The listing builds one solid part. Answer for the finished solid, in the listing's coordinates (mm). Face numbers are marked on the shaded views. A direction names the side the tool comes from. Give positions to 0.01 mm unless a question says otherwise; leave off trailing zeros. Write each loop counter-clockwise with the first axis right and the second up, starting at its lowest first coordinate (ties: lowest second). Pieces come first, ordered by that corner, then holes. Notation, with made-up numbers: (27.25, 3) - (68.25, 3) arc R22 ccw to (68.25, 15) - close; hole circle Ø2 at (72.25, 18). An arc over 180 degrees is marked (long way). Return JSON: item names as keys, results as strings.
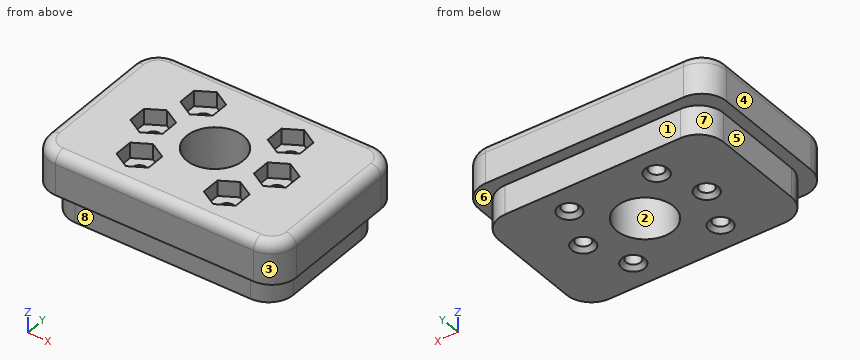
Autodesk Inventor part; units mm, degrees
ref_plane "Work Plane1" through (-0.635, 46.99, -50.8) normal (0, 1, 0) x (0, 0, 1)
ref_plane "YZ Plane" through (0, 0, 0) normal (1, 0, 0) x (0, 1, 0)
ref_plane "XZ Plane" through (0, 0, 0) normal (0, 1, 0) x (-1, 0, 0)
sketch "Sketch1" plane through (0, 0, 0) normal (0, 0, 1) x (1, 0, 0)
  line L0 (7.62, 0) -> (61.595, 0)
  line L1 (69.215, 7.62) -> (69.215, 36.195)
  line L2 (61.595, 43.815) -> (7.62, 43.815)
  line L3 (0, 36.195) -> (0, 7.62)
  arc A0 (7.62, 43.815) -> (0, 36.195) centre (7.62, 36.195) ccw
  arc A1 (0, 7.62) -> (7.62, 0) centre (7.62, 7.62) ccw
  arc A2 (61.595, 0) -> (69.215, 7.62) centre (61.595, 7.62) ccw
  arc A3 (69.215, 36.195) -> (61.595, 43.815) centre (61.595, 36.195) ccw
  point P0 (0, 0)
  point P1 (69.215, 43.815)
  point P2 (69.215, 0)
  point P3 (0, 43.815)
  dimension "d0" = 69.215
  dimension "d1" = 43.815
  dimension "d2" = 7.62
extrude "Extrusion1" add sketch "Sketch1" along normal blind 9
sketch "Sketch2" plane through (0, 0, 9) normal (0, 0, 1) x (1, 0, 0)
  line L0 (4.1275, -3.4925) -> (65.0875, -3.4925)
  line L1 (72.7075, 4.1275) -> (72.7075, 39.6875)
  line L2 (65.0875, 47.3075) -> (4.1275, 47.3075)
  line L3 (-3.4925, 39.6875) -> (-3.4925, 4.1275)
  arc A0 (4.1275, 47.3075) -> (-3.4925, 39.6875) centre (4.1275, 39.6875) ccw
  arc A1 (-3.4925, 4.1275) -> (4.1275, -3.4925) centre (4.1275, 4.1275) ccw
  arc A2 (65.0875, -3.4925) -> (72.7075, 4.1275) centre (65.0875, 4.1275) ccw
  arc A3 (72.7075, 39.6875) -> (65.0875, 47.3075) centre (65.0875, 39.6875) ccw
  line L4 (61.595, 43.815) -> (7.62, 43.815) construction
  line L5 (0, 36.195) -> (0, 7.62) construction
  point P0 (0, 0)
  point P1 (72.7075, 47.3075)
  point P2 (72.7075, -3.4925)
  point P3 (-3.4925, 47.3075)
  point P4 (34.6075, 47.3075)
  point P5 (34.6075, 43.815)
  point P6 (-3.4925, 21.9075)
  point P7 (0, 21.9075)
  dimension "d5" = 76.2
  dimension "d6" = 50.8
  dimension "d7" = 7.62
extrude "Extrusion2" add sketch "Sketch2" along normal blind 12.7
fillet "Fillet1" radius 3.175 8 edges at (-1.2607, 45.0757, 21.7) (-3.4925, 21.9075, 21.7) (-1.2607, -1.2607, 21.7) (34.6075, -3.4925, 21.7) (70.4757, -1.2607, 21.7) (72.7075, 21.9075, 21.7) (70.4757, 45.0757, 21.7) (34.6075, 47.3075, 21.7)
sketch "Sketch3" plane through (0, 0, 21.7) normal (0, 0, 1) x (1, 0, 0)
  line L0 (65.0875, 47.3075) -> (4.1275, 47.3075) construction
  line L1 (65.0875, 47.3075) -> (4.1275, 47.3075) construction
  line L2 (-3.4925, 39.6875) -> (-3.4925, 4.1275) construction
  line L3 (-3.4925, 39.6875) -> (-3.4925, 4.1275) construction
  circle A0 centre (34.6075, 21.9075) radius 8.75
  circle A1 centre (34.6075, 21.9075) radius 19 construction
  circle A2 centre (21.1725, 35.3425) radius 2.25
  circle A3 centre (48.0425, 35.3425) radius 2.25
  circle A4 centre (15.6075, 21.9075) radius 2.25
  circle A5 centre (53.6075, 21.9075) radius 2.25
  circle A6 centre (21.1725, 8.4725) radius 2.25
  circle A7 centre (48.0425, 8.4725) radius 2.25
  line L4 (21.1725, 35.3425) -> (34.6075, 21.9075) construction
  line L5 (34.6075, 21.9075) -> (15.6075, 21.9075) construction
  point P0 (0, 0)
  point P1 (34.6075, 47.3075)
  point P2 (-3.4925, 21.9075)
  point P3 (-3.4925, 21.9075)
  dimension "d11" = 17.5
  dimension "d14" = 4.5
  dimension "d15" = 38
  dimension "d16" = 45
extrude "Extrusion3" cut sketch "Sketch3" against normal up to surface (21.7 mm away)
chamfer "Chamfer1" distance 1.27 angle 45 6 edges at (45.7925, 35.3425, 0) (18.9225, 35.3425, 0) (13.3575, 21.9075, 0) (51.3575, 21.9075, 0) (45.7925, 8.4725, 0) (18.9225, 8.4725, 0)
sketch "Sketch4" plane through (7.62, 0, 0) normal (0, -1, 0) x (1, 0, 0)
  point P0 (-7.62, 0)
ref_plane "Work Plane1" through (-0.635, 46.99, -50.8) normal (0, 1, 0) x (0, 0, 1)
sketch "Sketch7" plane through (0, 0, 21.7) normal (0, 0, 1) x (1, 0, 0)
  line L0 (21.1725, 2.7532) -> (16.2195, 5.6129)
  line L1 (16.2195, 5.6129) -> (16.2195, 11.3321)
  line L2 (16.2195, 11.3321) -> (21.1725, 14.1917)
  line L3 (21.1725, 14.1917) -> (26.1255, 11.3321)
  line L4 (26.1255, 11.3321) -> (26.1255, 5.6129)
  line L5 (26.1255, 5.6129) -> (21.1725, 2.7532)
  circle A0 centre (48.0425, 35.3425) radius 2.25 construction
  circle A1 centre (53.6075, 21.9075) radius 2.25 construction
  circle A2 centre (48.0425, 8.4725) radius 2.25 construction
  circle A3 centre (21.1725, 8.4725) radius 2.25 construction
  circle A4 centre (15.6075, 21.9075) radius 2.25 construction
  circle A5 centre (21.1725, 35.3425) radius 2.25 construction
  line L6 (53.6075, 16.1883) -> (48.6545, 19.0479)
  line L7 (48.6545, 19.0479) -> (48.6545, 24.7671)
  line L8 (48.6545, 24.7671) -> (53.6075, 27.6267)
  line L9 (53.6075, 27.6267) -> (58.5605, 24.7671)
  line L10 (58.5605, 24.7671) -> (58.5605, 19.0479)
  line L11 (58.5605, 19.0479) -> (53.6075, 16.1883)
  line L12 (48.0425, 29.6233) -> (43.0895, 32.4829)
  line L13 (43.0895, 32.4829) -> (43.0895, 38.2021)
  line L14 (43.0895, 38.2021) -> (48.0425, 41.0618)
  line L15 (48.0425, 41.0618) -> (52.9955, 38.2021)
  line L16 (52.9955, 38.2021) -> (52.9955, 32.4829)
  line L17 (52.9955, 32.4829) -> (48.0425, 29.6233)
  line L18 (15.6075, 16.1883) -> (10.6545, 19.0479)
  line L19 (10.6545, 19.0479) -> (10.6545, 24.7671)
  line L20 (10.6545, 24.7671) -> (15.6075, 27.6267)
  line L21 (15.6075, 27.6267) -> (20.5605, 24.7671)
  line L22 (20.5605, 24.7671) -> (20.5605, 19.0479)
  line L23 (20.5605, 19.0479) -> (15.6075, 16.1883)
  line L24 (21.1725, 29.6233) -> (16.2195, 32.4829)
  line L25 (16.2195, 32.4829) -> (16.2195, 38.2021)
  line L26 (16.2195, 38.2021) -> (21.1725, 41.0618)
  line L27 (21.1725, 41.0618) -> (26.1255, 38.2021)
  line L28 (26.1255, 38.2021) -> (26.1255, 32.4829)
  line L29 (26.1255, 32.4829) -> (21.1725, 29.6233)
  line L30 (48.0425, 2.7532) -> (43.0895, 5.6129)
  line L31 (43.0895, 5.6129) -> (43.0895, 11.3321)
  line L32 (43.0895, 11.3321) -> (48.0425, 14.1917)
  line L33 (48.0425, 14.1917) -> (52.9955, 11.3321)
  line L34 (52.9955, 11.3321) -> (52.9955, 5.6129)
  line L35 (52.9955, 5.6129) -> (48.0425, 2.7532)
  point P0 (0, 0)
  dimension "d26" = 9.906
extrude "Extrusion6" cut sketch "Sketch7" against normal blind 4.7625
properties part number "2x3_Spacer_Rear"
Item 1: Flat-ended cylindrical pins translate along their axes: P1, Ø2, axis at y = 7, z = 3, coming from the -X side; P2, Ø5, axis at x = 48.04, y = 8.47, coming from the -Z side; P3, Ø4.5, axis at x = 25, z = 3, coming from the -Y side. Find the tip coordinate at first contact, or state that the pin passes through.
Answer below:
{"P1": "stops at x = 0", "P2": "stops at z = 1.02", "P3": "stops at y = 0"}
Item 2: For the marked faces 5, 6, 7 and 8, determine the directions among +Z, -Z, +X, -X, +Y, -Y from which every point of the face is accessible in a straight line to the end or side of a thin tool.
Answer below:
{"face 5": "-Z, -X, +Y, -Y", "face 6": "-Z", "face 7": "-Z, -X, +Y", "face 8": "-Z, +X, -X, -Y"}
Item 3: Consider L1, parallel to X at y = 13, z = 19.25; L2, parallel to X at y = 21, z = 3.5 (3 decimals); L3, parallel to X at y = 8, z = 16.25. Determine where each line is inside the solid, lowest interval first.
Answer below:
{"L1": "x = -3.41 to 19.11, 23.24 to 45.98, 50.11 to 72.62", "L2": "x = 0 to 13.549, 17.666 to 25.905, 43.31 to 51.549, 55.666 to 69.215", "L3": "x = -3.49 to 18.97, 23.37 to 45.84, 50.24 to 72.71"}
Item 4: A cutting plane is placed at C-C on z = 10. Determine the outline of the cut face in (x, y).
Answer below:
{"outline": "(-3.49, 4.13) arc R7.62 ccw to (4.13, -3.49) - (65.09, -3.49) arc R7.62 ccw to (72.71, 4.13) - (72.71, 39.69) arc R7.62 ccw to (65.09, 47.31) - (4.13, 47.31) arc R7.62 ccw to (-3.49, 39.69) - close; hole circle Ø4.5 at (15.61, 21.91); hole circle Ø4.5 at (21.17, 8.47); hole circle Ø4.5 at (21.17, 35.34); hole circle Ø17.5 at (34.61, 21.91); hole circle Ø4.5 at (48.04, 8.47); hole circle Ø4.5 at (48.04, 35.34); hole circle Ø4.5 at (53.61, 21.91)"}
Item 5: The mould has two halves that part along Y. Classify the marked faces 1, 2, 3 and 4: +Y half, -Y half, draft (parallel to the pull), parting line (faces both ways), or undercut.
Answer below:
{"face 1": "+Y half", "face 2": "undercut", "face 3": "-Y half", "face 4": "draft"}
